from build123d import *

# Parameters (mm, degrees)
SKETCH1_R                         = 12.7
BOSS_EXTRUDE1_DEPTH               = 79.375
SKETCH2_R                         = 21.293421543
SKETCH2_R_2                       = 9.525
CUT_EXTRUDE1_DEPTH                = 19.05
SKETCH3_W                         = 88.347660667
SKETCH3_H                         = 62.084650607
CUT_EXTRUDE2_DEPTH                = 7.62
SKETCH7_W                         = 118.824828897
SKETCH7_H                         = 51.847980611
CUT_EXTRUDE5_DEPTH                = 25.4
F_1_4_20_TAPPED_HOLE2_D           = 5.1054
F_1_4_20_TAPPED_HOLE2_DEPTH       = 16.002
F_1_4_20_TAPPED_HOLE2_CSINK_D     = 7.112
F_1_4_20_TAPPED_HOLE2_CSINK_ANGLE = 82
F_1_4_20_TAPPED_HOLE2_TIP         = 1.533816902
F_1_4_20_TAPPED_HOLE3_D           = 5.1054
F_1_4_20_TAPPED_HOLE3_DEPTH       = 16.002
F_1_4_20_TAPPED_HOLE3_CSINK_D     = 7.112
F_1_4_20_TAPPED_HOLE3_CSINK_ANGLE = 82
F_1_4_20_TAPPED_HOLE3_TIP         = 1.533816902
CUT_EXTRUDE10_DEPTH               = 88.9
SKETCH18_R                        = 21.68820387
CUT_EXTRUDE12_DEPTH               = 3.175
SKETCH30_R                        = 17.847306034
SKETCH30_R_2                      = 9.525
CUT_EXTRUDE13_DEPTH               = 19.05
F_1_4_20_TAPPED_HOLE6_D           = 5.1054
F_1_4_20_TAPPED_HOLE6_DEPTH       = 16.002
F_1_4_20_TAPPED_HOLE6_CSINK_D     = 7.112
F_1_4_20_TAPPED_HOLE6_CSINK_ANGLE = 82
F_1_4_20_TAPPED_HOLE6_TIP         = 1.533816902
F_1_4_20_TAPPED_HOLE7_D           = 5.1054
F_1_4_20_TAPPED_HOLE7_DEPTH       = 16.002
F_1_4_20_TAPPED_HOLE7_CSINK_D     = 7.112
F_1_4_20_TAPPED_HOLE7_CSINK_ANGLE = 82
F_1_4_20_TAPPED_HOLE7_TIP         = 1.533816902


with BuildPart() as part:
    # Sketch1 → Boss-Extrude1 (new body)
    with BuildSketch(Plane(origin=(0, 0, 0), x_dir=(0, 0, -1), z_dir=(1, 0, 0))):
        Circle(SKETCH1_R)
    extrude(amount=-BOSS_EXTRUDE1_DEPTH)

    # Sketch2 → Cut-Extrude1 (cut)
    with BuildSketch(Plane(origin=(0, 0, 0), x_dir=(0, 0, -1), z_dir=(1, 0, 0))):
        Circle(SKETCH2_R)
        Circle(SKETCH2_R_2, mode=Mode.SUBTRACT)
    extrude(amount=-CUT_EXTRUDE1_DEPTH, mode=Mode.SUBTRACT)

    # Sketch3 → Cut-Extrude2 (cut)
    with BuildSketch(Plane(origin=(0, 12.401228443, 11.1252), x_dir=(1, 0, 0), z_dir=(0, 0, 1))):
        with Locations((-47.069787049, -6.880973923)):
            Rectangle(SKETCH3_W, SKETCH3_H)
    extrude(amount=CUT_EXTRUDE2_DEPTH, mode=Mode.SUBTRACT)

    # Sketch7 → Cut-Extrude5 (cut)
    with BuildSketch(Plane(origin=(0, 11.1252, 0), x_dir=(-1, 0, 0), z_dir=(0, 1, 0))):
        with Locations((37.000899043, -1.114295637)):
            Rectangle(SKETCH7_W, SKETCH7_H)
    extrude(amount=CUT_EXTRUDE5_DEPTH, mode=Mode.SUBTRACT)

    # 1/4-20 Tapped Hole2
    with Locations(Plane(origin=(0, 11.1252, 0), x_dir=(-1, 0, 0), z_dir=(0, 1, 0))):
        with Locations((25.4, 0)):
            CounterSinkHole(F_1_4_20_TAPPED_HOLE2_D / 2, F_1_4_20_TAPPED_HOLE2_CSINK_D / 2, depth=F_1_4_20_TAPPED_HOLE2_DEPTH, counter_sink_angle=F_1_4_20_TAPPED_HOLE2_CSINK_ANGLE)
            with Locations((0, 0, -(F_1_4_20_TAPPED_HOLE2_DEPTH + F_1_4_20_TAPPED_HOLE2_TIP / 2))):  # 118° drill point
                Cone(0, F_1_4_20_TAPPED_HOLE2_D / 2, F_1_4_20_TAPPED_HOLE2_TIP, mode=Mode.SUBTRACT)

    # 1/4-20 Tapped Hole3
    with Locations(Plane(origin=(0, 0, 0), x_dir=(0, 0, -1), z_dir=(1, 0, 0))):
        with Locations((0, 0)):
            CounterSinkHole(F_1_4_20_TAPPED_HOLE3_D / 2, F_1_4_20_TAPPED_HOLE3_CSINK_D / 2, depth=F_1_4_20_TAPPED_HOLE3_DEPTH, counter_sink_angle=F_1_4_20_TAPPED_HOLE3_CSINK_ANGLE)
            with Locations((0, 0, -(F_1_4_20_TAPPED_HOLE3_DEPTH + F_1_4_20_TAPPED_HOLE3_TIP / 2))):  # 118° drill point
                Cone(0, F_1_4_20_TAPPED_HOLE3_D / 2, F_1_4_20_TAPPED_HOLE3_TIP, mode=Mode.SUBTRACT)

    # Sketch26 → Cut-Extrude10 (cut)
    with BuildSketch(Plane(origin=(0, 0, 0), x_dir=(0, 0, -1), z_dir=(1, 0, 0))):
        Polygon((-14.121239211, -11.1252), (11.1252, -11.1252), (11.1252, 12.077626787), (19.494279453, 12.077626787), (19.494279453, -11.628277338), (15.190001849, -11.628277338), (15.190001849, -15.796314113), (-14.121239211, -15.796314113), align=None)
    extrude(amount=-CUT_EXTRUDE10_DEPTH, mode=Mode.SUBTRACT)

    # Sketch18 → Cut-Extrude12 (cut)
    with BuildSketch(Plane.ZY.offset(79.375)):
        Circle(SKETCH18_R)
    extrude(amount=-CUT_EXTRUDE12_DEPTH, mode=Mode.SUBTRACT)

    # Sketch30 → Cut-Extrude13 (cut)
    with BuildSketch(Plane.ZY.offset(76.2)):
        Circle(SKETCH30_R)
        Circle(SKETCH30_R_2, mode=Mode.SUBTRACT)
    extrude(amount=-CUT_EXTRUDE13_DEPTH, mode=Mode.SUBTRACT)

    # 1/4-20 Tapped Hole6
    with Locations(Plane.ZY.offset(76.2)):
        with Locations((0, 0)):
            CounterSinkHole(F_1_4_20_TAPPED_HOLE6_D / 2, F_1_4_20_TAPPED_HOLE6_CSINK_D / 2, depth=F_1_4_20_TAPPED_HOLE6_DEPTH, counter_sink_angle=F_1_4_20_TAPPED_HOLE6_CSINK_ANGLE)
            with Locations((0, 0, -(F_1_4_20_TAPPED_HOLE6_DEPTH + F_1_4_20_TAPPED_HOLE6_TIP / 2))):  # 118° drill point
                Cone(0, F_1_4_20_TAPPED_HOLE6_D / 2, F_1_4_20_TAPPED_HOLE6_TIP, mode=Mode.SUBTRACT)

    # 1/4-20 Tapped Hole7
    with Locations(Plane.XZ.offset(11.1252)):
        with Locations((-50.8, 0)):
            CounterSinkHole(F_1_4_20_TAPPED_HOLE7_D / 2, F_1_4_20_TAPPED_HOLE7_CSINK_D / 2, depth=F_1_4_20_TAPPED_HOLE7_DEPTH, counter_sink_angle=F_1_4_20_TAPPED_HOLE7_CSINK_ANGLE)
            with Locations((0, 0, -(F_1_4_20_TAPPED_HOLE7_DEPTH + F_1_4_20_TAPPED_HOLE7_TIP / 2))):  # 118° drill point
                Cone(0, F_1_4_20_TAPPED_HOLE7_D / 2, F_1_4_20_TAPPED_HOLE7_TIP, mode=Mode.SUBTRACT)


solid = part.part
Input: part model. Units: mm. Frame: model coordinates. A direction names the side the tool comes from. Coordinates: 2 decimals unless noted, no trailing zeros. Loops run counter-clockwise (first coordinate to the right, second up) from the corner with the lowest first, then second, coordinate; pieces in that order, holes last.
Q1. Cut plane A-A (y = 8.5). Output: boundary loops of the cut face in (x, z).
Q2. Set-up query: faces 1 (the face through (-48.25, -2.44, 0.11)), 2 (the face through (-25.81, -6.144, -0.17)), 3 (the face through (-76.2, 0, 4)), 4 (the face through (-19.05, -10, 0)), 5 (the face through (-57.15, 0, 10)). Return all of +Z, -Z, +X, -X, +Y, -Y with unobstructed straight access to the full face (end or side cutting, diameter ignored); none if empty.
Q3. Material intervals for line 1 (X direction, y = -4, z = 0); line 2 (Z direction, x = -50.8, y = -2.75); line 3 (Y direction, x = -9.75, z = 0) (3 decimals), sorted ascending.
Q4. Draft query along Y for faces 6 (the face through (-8.682, 0.767, 2.435)), 7 (the face through (-37.83, -8.94, 9.02)), 8 (the face through (-37.83, 8.94, -9.02)). Return one class per face: +Y half, -Y half, draft (parallel to the pull), parting line (faces both ways), or undercut.
Q5. Cut plane B-B (x = -9). Output: boundary loops of the cut face in (y, z) (3 decimals).
Q6. Cut plane C-C (y = -0.75). Give the number of separate pieces and of enclosed holes in the cut face, then the cut area to 3 significant figures.
Q7. Contact query for flat-ended pins moving along their axis: pin 1 (8 mm diameter, centred on x = -63.5, y = 0.5, fed in from +Z) (3 decimals); pin 2 (4 mm diameter, centred on x = -25.4, z = 0, fed in from +Y); pin 3 (1 mm diameter, centred on x = -57.5, y = -9, fed in from -Z). Output: stop coordinate, or through.
Working result:
1. outline: (-76.2, -4.3) - (-57.15, -4.3) - (-57.15, -9.44) - (-19.05, -9.44) - (-19.05, -4.3) - (0, -4.3) - (0, 4.3) - (-19.05, 4.3) - (-19.05, 9.44) - (-57.15, 9.44) - (-57.15, 4.3) - (-76.2, 4.3) - close; hole circle Ø5.11 at (-25.4, 0)
2. face 1: -Y
2. face 2: +Y
2. face 3: +Z, -Z, -X, +Y, -Y
2. face 4: +X
2. face 5: -X
3. line 1: x = -76.2 to -53.35, -48.25 to -27.95, -22.85 to 0
3. line 2: z = -11.13 to -2.55, 2.55 to 11.13
3. line 3: y = -9.525 to -2.553, 2.553 to 9.525
4. face 6: undercut
4. face 7: -Y half
4. face 8: +Y half
5. outline: circle Ø19.05 at (0, 0); hole circle Ø5.105 at (0, 0)
6. separate pieces: 1
6. enclosed holes: 2
6. area: 1,370 mm2
7. pin 1: stops at z = 9.525
7. pin 2: stops at y = -5.21
7. pin 3: stops at z = -9.31
